The model under review builds one solid part; all positions refer to its coordinate system, in mm. Face numbers are marked on the shaded views. A direction names the side the tool comes from. Round coordinates to 2 decimals unless told otherwise and drop trailing zeros. Write each loop counter-clockwise with the first axis right and the second up, starting at its lowest first coordinate (ties: lowest second). Pieces come first, ordered by that corner, then holes. Notation, with made-up numbers: M -33.5,-32.5 L -5.5,-32.5 A8 cw -5.5,-24.5 Z; hole C 46.25,10 d11. An arc over 180 degrees is marked long. Write item = value, one per line. Start each with the question number.
Item 1: Tool access review of the marked faces 1, 2, 3, 4 and 5: name each direction out of +Z, -Z, +X, -X, +Y, -Y from which nothing blocks a thin tool from reaching the whole face with its end or side.
Item 2: The part is to be moulded in two halves that separate along Y. For the marked faces 6, 7 and 8, say which applies: +Y half, -Y half, draft (parallel to the pull), parting line (faces both ways), or undercut.
Item 3: Take a section at C-C, the plane y = -9. Give the boundary of the cut face in (x, z), plus the area to 3 significant figures.
Item 4: Take a section at D-D, the plane z = 10.5. Give the boundary of the cut face in (x, y).
Item 5: Take a section at A-A, the plane y = 0. Give the boundary of the cut face in (x, z).
Item 6: To check wall thickness, follow line 1 along Y through (x, z) = (0, 5.5); line 2 along Y through (x, z) = (0, 12.6); line 3 along Z through (x, y) = (-8, -6.5). State the ranges of each line that lie inside material, in increasing order.
Item 7: For pin 1 Ø4 at (x, z) = (2.5, 1.5) entering from +Y; pin 2 Ø6 at (x, z) = (4, 13) entering from +Y; pin 3 Ø7 at (x, y) = (-1, -0.5) entering from -Z; pin 4 Ø11.5 at (x, y) = (-1.5, 2.5) entering from -Z, all flat-tipped, find the tip position at first contact; note any pin that passes through.
Autodesk Inventor part; units mm, degrees
ref_plane "YZ Plane" through (0, 0, 0) normal (1, 0, 0) x (0, 1, 0)
ref_plane "XZ Plane" through (0, 0, 0) normal (0, 1, 0) x (-1, 0, 0)
ref_plane "XY Plane" through (0, 0, 0) normal (0, 0, 1) x (1, 0, 0)
sketch "スケッチ1" plane through (0, 0, 0) normal (0, 0, 1) x (1, 0, 0)
  circle A0 centre (0, 0) radius 10
  dimension "d0" = 20
extrude "押し出し1" add sketch "スケッチ1" along normal blind 6
sketch "スケッチ2" plane through (0, 0, 0) normal (0, 0, -1) x (-1, 0, 0)
  circle A0 centre (0, 0) radius 12
  circle A1 centre (0, 0) radius 10
  dimension "d17" = 2
extrude "押し出し2" add sketch "スケッチ2" along normal blind 3 contours A0 | A1
sketch "スケッチ3" plane through (0, 0, -3) normal (0, 0, -1) x (-1, 0, 0)
  circle A0 centre (0, 0) radius 8
  dimension "d6" = 16
hole "穴1" at (0, 0, -3) direction (0, 0, 1) diameter 8.4 end through all
sketch "スケッチ4" plane through (0, 0, -3) normal (0, 0, -1) x (-1, 0, 0)
  circle A0 centre (0, 0) radius 7.1
  dimension "d14" = 14.2
extrude "押し出し3" cut sketch "スケッチ4" against normal blind 3.4
mirror "ミラー1" about plane through (0, 0, 6) normal (0, 0, 1) of "押し出し1", "押し出し2", "穴1", "押し出し3"
fillet "フィレット1" radius 1 2 edges at (7.1, 0, 15) (7.1, 0, -3)
properties part number "link1part5"
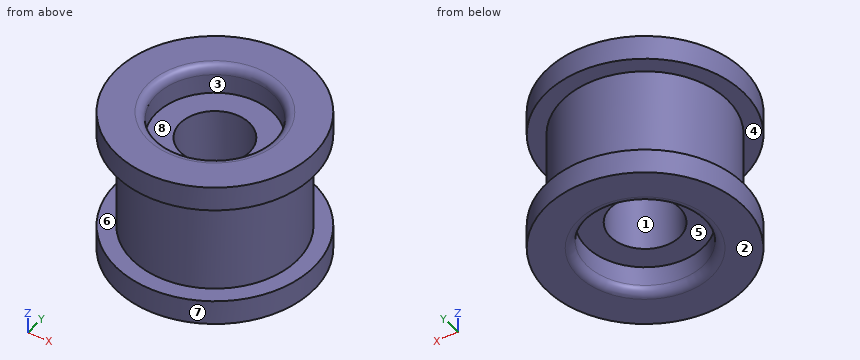
Response values:
q1.face_1 = +Z, -Z
q1.face_2 = -Z, +X, -X, +Y, -Y
q1.face_3 = +Z
q1.face_4 = none
q1.face_5 = -Z
q2.face_6 = draft
q2.face_7 = parting line
q2.face_8 = undercut
q3.outline = M -7.94,-3 L 7.94,-3 L 7.94,0 L 4.36,0 L 4.36,12 L 7.94,12 L 7.94,15 L -7.94,15 L -7.94,12 L -4.36,12 L -4.36,0 L -7.94,0 Z
q3.area = 200 mm2
q4.outline = C 0,0 d20; hole C 0,0 d8.4
q5.outline = M -12,-3 L -8.1,-3 A1 ccw -7.1,-2 L -7.1,0.4 L -4.2,0.4 L -4.2,11.6 L -7.1,11.6 L -7.1,14 A1 ccw -8.1,15 L -12,15 L -12,12 L -10,12 L -10,0 L -12,0 Z; M 4.2,0.4 L 7.1,0.4 L 7.1,-2 A1 ccw 8.1,-3 L 12,-3 L 12,0 L 10,0 L 10,12 L 12,12 L 12,15 L 8.1,15 A1 ccw 7.1,14 L 7.1,11.6 L 4.2,11.6 Z
q6.line_1 = -10 to -4.2, 4.2 to 10
q6.line_2 = -12 to -7.1, 7.1 to 12
q6.line_3 = -3 to 0, 12 to 15
q7.pin_1 = 11.94
q7.pin_2 = 11.96
q7.pin_3 = 0.4
q7.pin_4 = -3
